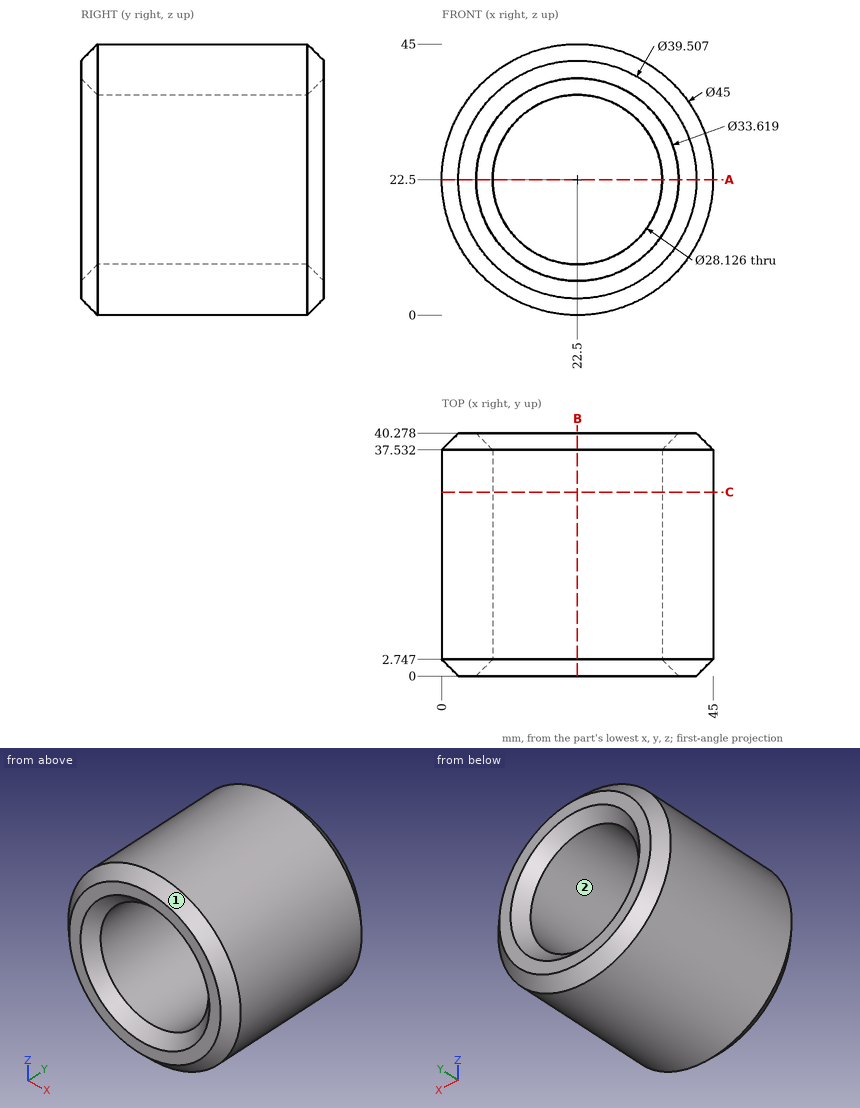
Geometry: see drawing. Coordinates: mm, zero at the bounding-box minimum. Give positions to 0.01 mm unless a question says otherwise; leave off trailing zeros. Order: outer loops, then holes, each group sorted by start corner. A loop starts at its lowest first (then second) coordinate and runs counter-clockwise, first axis right, second up. Notation, with made-up numbers: (69, 68) - (90, 68) arc R26 ccw to (90, 89) - close; hole circle Ø6 at (-22.75, 18). An arc over 180 degrees is marked (long way). Write each question's results on one line, items separated by ' | '.
Item 1: Material intervals for line 1 along X through (y, z) = (20.5, 22.5); line 2 along Z through (x, y) = (23, 19.5) (1 decimal); line 3 along Z through (x, y) = (32.5, 4) (1 decimal), sorted ascending.
A:
line 1: x = 0 to 8.44, 36.56 to 45 | line 2: z = 0 to 8.4, 36.6 to 45 | line 3: z = 2.3 to 12.6, 32.4 to 42.7
Item 2: Section A-A (z = 22.5). Return loops of the section in (x, y).
A:
outline: (0, 2.75) - (2.75, 0) - (5.69, 0) - (8.44, 2.75) - (8.44, 37.53) - (5.69, 40.28) - (2.75, 40.28) - (0, 37.53) - close; (36.56, 2.75) - (39.31, 0) - (42.25, 0) - (45, 2.75) - (45, 37.53) - (42.25, 40.28) - (39.31, 40.28) - (36.56, 37.53) - close
Item 3: Contact query for flat-ended pins moving along their axis: pin 1 Ø12 at (x, z) = (28, 27) entering from -Y; pin 2 Ø12 at (x, y) = (12, 15.5) entering from +Z (1 decimal); pin 3 Ø4 at (y, z) = (11.5, 13) entering from +X; pin 4 Ø8 at (y, z) = (20.5, 18.5) entering from -X. Output: stop coordinate, or through.
A:
pin 1: passes through | pin 2: stops at z = 44.5 | pin 3: stops at x = 43.71 | pin 4: stops at x = 0
Item 4: Section B-B (x = 22.5). Return loops of the section in (y, z).
A:
outline: (0, 2.75) - (2.75, 0) - (37.53, 0) - (40.28, 2.75) - (40.28, 5.69) - (37.53, 8.44) - (2.75, 8.44) - (0, 5.69) - close; (0, 39.31) - (2.75, 36.56) - (37.53, 36.56) - (40.28, 39.31) - (40.28, 42.25) - (37.53, 45) - (2.75, 45) - (0, 42.25) - close
Item 5: Draft query along X for the marked faces 1 and 2. Return one class per face: released by +X, released by -X, zero draft, split by the parting line, or undercut.
A:
face 1: split by the parting line | face 2: undercut
Item 6: Section C-C (y = 30.5). Return loops of the section in (x, z) (1 decimal), and give its area (3 significant figures).
A:
outline: circle Ø45 at (22.5, 22.5); hole circle Ø28.1 at (22.5, 22.5) | area: 969 mm^2
